Autodesk Fusion 360 part; units mm, degrees
sketch "Sketch1" plane through (0, 0, 0) normal (0, 0, 1) x (1, 0, 0)
  line L0 (0, 0) -> (-78, 0)
  line L1 (-78, 0) -> (-78, 22)
  line L2 (-78, 22) -> (0, 22)
  line L3 (0, 22) -> (0, 0)
  dimension "d1" = 78
  dimension "d2" = 22
extrude "Extrude1" add sketch "Sketch1" along normal blind 2
sketch "Sketch2" plane through (0, 0, 0) normal (1, 0, 0) x (0, 1, 0)
  line L0 (0, 0) -> (22, 0)
  line L1 (22, 0) -> (22, 2)
  line L2 (22, 2) -> (0, 2)
  line L3 (0, 2) -> (0, 0)
  line L4 (0, 2) -> (0, 20)
  line L5 (0, 20) -> (22, 20)
  line L6 (22, 20) -> (22, 2)
  circle A0 centre (11, 20) radius 7.5
  dimension "d8" = 18
  dimension "d9" = 15
extrude "Extrude2" add sketch "Sketch2" against normal blind 3 contours L2 L4 L5 L6 A0
sketch "Sketch3" plane through (-78, 0, 0) normal (-1, 0, 0) x (0, -1, 0)
  line L0 (-22, 0) -> (0, 0)
  line L1 (0, 0) -> (0, 2)
  line L2 (0, 2) -> (-22, 2)
  line L3 (-22, 2) -> (-22, 0)
  line L4 (0, 0) -> (-22, 0)
  line L5 (-22, 0) -> (-22, 2)
  line L6 (-22, 2) -> (0, 2)
  line L7 (0, 2) -> (0, 0)
  line L8 (0, 2) -> (0, 20)
  line L9 (0, 20) -> (-22, 20)
  line L10 (-22, 20) -> (-22, 2)
  circle A0 centre (-11, 20) radius 1.7
  dimension "d12" = 3.4
extrude "Extrude3" add sketch "Sketch3" against normal blind 3 contours L2 L6 L8 L9 L10 A0
fillet "Fillet1" radius 4 2 edges at (-75, 11, 2) (-3, 11, 2)
equation "d1 = 81 mm - 3 mm"
Work out the finished part from the listing and answer in its coordinate system (mm). A direction names the side the tool comes from. Round coordinates to 2 decimals unless told otherwise and drop trailing zeros. Write each loop counter-clockwise with the first axis right and the second up, starting at its lowest first coordinate (ties: lowest second). Pieces come first, ordered by that corner, then holes. Notation, with made-up numbers: (-34.75, -3.5) -> (-15.75, -3.5) arc R22 cw to (-15.75, 28.5) -> close; hole circle Ø7 at (-37, -5). An arc over 180 degrees is marked (long way). Answer as CSV lines item,"result". Start each with the question number.
(1) The part is cut by section A-A, the plane z = 8.25. Give the vertices of the cut face in (x, y).
(2) A tool of negligible diameter and unlimited length cuts with its end or side. For faces 5 (the flat face through (-75, 11, 13)), 6 (the flat face through (-77, 17, 20)), 7 (the cylindrical face through (-1.48, 10.84, 12.5)), from which of +Z, -Z, +X, -X, +Y, -Y can it reach the whole face along a straight path? Write none if from no direction.
(3) The mould has two halves that part along X. Classify faces 1 (the flat face through (-3, 11, 12)), 2 (the flat face through (0, 11, 8)), 3 (the cylindrical face through (-4.203, 10.846, 3.141)), 4 (the flat face through (-1, 2, 20)): +X half, -X half, draft (parallel to the pull), parting line (faces both ways), or undercut.
(4) This flat-tipped pin is pushed along its axis until it touches: pin 1 (4 mm diameter, centred on x = -69.5, y = 6, fed in from +Z). Where does it stop, or does it pass through?
(5) The part is cut by section C-C, the plane z = 13.5. Give the vertices of the cut face in (x, y).
(6) Find the intervals of material crossed by probe 1 along X at (y, z) = (18.25, 12); probe 2 along Z at (x, y) = (-23.5, 16.25); probe 3 along X at (y, z) = (4.25, 3.5), in increasing order.
(7) The part is cut by section B-B, the plane y = 11. Give the vertices of the cut face in (x, z).
(8) The part is cut by section D-D, the plane x = -19.5. Give the vertices of the cut face in (y, z), then the cut area to 3 significant figures.
Output values:
1,outline,"(-78, 0) -> (-75, 0) -> (-75, 22) -> (-78, 22) -> close; (-3, 0) -> (0, 0) -> (0, 22) -> (-3, 22) -> close"
2,face 5,"+Z, +Y, -Y"
2,face 6,"+Z, +X, -X, +Y, -Y"
2,face 7,"+Z, +X"
3,face 1,"undercut"
3,face 2,"+X half"
3,face 3,"undercut"
3,face 4,"draft"
4,pin 1,"stops at z = 2.03"
5,outline,"(-78, 0) -> (-75, 0) -> (-75, 22) -> (-78, 22) -> close; (-3, 0) -> (0, 0) -> (0, 7.26) -> (-3, 7.26) -> close; (-3, 14.74) -> (0, 14.74) -> (0, 22) -> (-3, 22) -> close"
6,probe 1,"x = -78 to -75, -3 to 0"
6,probe 2,"z = 0 to 2"
6,probe 3,"x = -78 to -74.12, -3.88 to 0"
7,outline,"(-78, 0) -> (0, 0) -> (0, 12.5) -> (-3, 12.5) -> (-3, 6) arc R4 cw to (-7, 2) -> (-71, 2) arc R4 cw to (-75, 6) -> (-75, 18.3) -> (-78, 18.3) -> close"
8,outline,"(0, 0) -> (22, 0) -> (22, 2) -> (0, 2) -> close"
8,area,"44.0 mm²"
